Verification items for the finished model (mm, model axes). A direction names the side the tool comes from. Coordinates: 2 decimals unless noted, no trailing zeros. Order: outer loops, then holes, each group sorted by start corner. A loop starts at its lowest first (then second) coordinate and runs counter-clockwise, first axis right, second up.
Q1. Thickness scan on line 1 (Z direction, x = -11, y = 29.5); line 2 (Z direction, x = 8.5, y = -4); line 3 (Y direction, x = 0, z = 23). Record the ranges inside material, lowest first.
Q2. Cross-section at B-B, the plane z = 15. Record the boundary of the cut face in (x, y), and give its area (3 significant figures).
Q3. Set-up check for faces 1 (the flat face through (2, 5, -4)), 2 (the cylindrical face through (-42.15, -41.99, 16.78)): record each of +Z, -Z, +X, -X, +Y, -Y from which the full face is reachable in a straight line by a thin tool's end or side.
Q4. Depth check by flat-ended pin: P1, Ø13, axis at x = 0, y = 0, coming from the -Z side; P2, Ø12, axis at y = -24.5, z = -19.5, coming from the +X side; P3, Ø8, axis at y = 7.5, z = -5.5, coming from the -X side. Enter the tip coordinate at first touch or a pass-through.
Q5. Draft check along Y on faces 3 (the flat face through (0, 45, 16)), 4 (the cylindrical face through (-1.08, -4.88, 16.32)), 5 (the flat face through (-1, 21, 0)). Enter one of: pulls with the +Y half, pulls with the -Y half, needs draft (parallel to the pull), parting line crosses it, or undercut.
Q6. Cross-section at C-C, the plane x = 0. Record the boundary of the cut face in (y, z), and give its area (3 significant figures).
Q7. Cross-section at D-D, the plane y = 0. Record the boundary of the cut face in (x, z).
Q8. Cross-section at A-A, the plane y = 32. Record the boundary of the cut face in (x, z).
from build123d import *

# Parameters (mm, degrees)
SKETCH1_W                               = 40
SKETCH1_H                               = 19.3
SKETCH2_R                               = 20
BOSS_EXTRUDE1_DEPTH                     = 6.5
CBORE_FOR_M8_HEX_HEAD_BOLT1_D           = 10
CBORE_FOR_M8_HEX_HEAD_BOLT1_CBORE_D     = 20
CBORE_FOR_M8_HEX_HEAD_BOLT1_CBORE_DEPTH = 4
F_5_0_5_DIAMETER_HOLE1_D                = 5
F_5_0_5_DIAMETER_HOLE1_DEPTH            = 8
SKETCH7_W                               = 90
SKETCH7_H                               = 90
SKETCH7_R                               = 5
BOSS_EXTRUDE2_DEPTH                     = 33.1
FILLET1_R                               = 10


with BuildPart() as part:
    # Sketch1 → Revolve1 (revolve)
    with BuildSketch(Plane.XZ, mode=Mode.PRIVATE) as revolve1_sk:
        with Locations((20, -16.15)):
            Rectangle(SKETCH1_W, SKETCH1_H)
    revolve(revolve1_sk.sketch.rotate(Axis((0, 0, -6.5), (0, 0, -1)), 270), axis=Axis((0, 0, -6.5), (0, 0, -1)))

    # Sketch2 → Boss-Extrude1 (add)
    with BuildSketch(Plane.XY.offset(-6.5)):
        Circle(SKETCH2_R)
    extrude(amount=BOSS_EXTRUDE1_DEPTH)

    # CBORE for M8 Hex Head Bolt1 (through all)
    with Locations(Plane.XY):
        with Locations((0, 0)):
            CounterBoreHole(CBORE_FOR_M8_HEX_HEAD_BOLT1_D / 2, CBORE_FOR_M8_HEX_HEAD_BOLT1_CBORE_D / 2, CBORE_FOR_M8_HEX_HEAD_BOLT1_CBORE_DEPTH)

    # Ø5.0 (5) Diameter Hole1
    with Locations(Plane.XY):
        with Locations((-15.75, 0), (-11.136931804, 11.136931804), (-11.136931804, -11.136931804), (11.136931804, -11.136931804), (11.136931804, 11.136931804)):
            Hole(F_5_0_5_DIAMETER_HOLE1_D / 2, depth=F_5_0_5_DIAMETER_HOLE1_DEPTH)

    # Sketch7 → Boss-Extrude2 (add)
    with BuildSketch(Plane.XY):
        Rectangle(SKETCH7_W, SKETCH7_H)
        Circle(SKETCH7_R, mode=Mode.SUBTRACT)
    extrude(amount=BOSS_EXTRUDE2_DEPTH)

    # Fillet1
    fillet1_edges = [part.edges().sort_by_distance(p)[0] for p in [
        (45, -45, 16.55),
        (45, 45, 16.55),
        (-45, 45, 16.55),
        (-45, -45, 16.55),
    ]]
    fillet(fillet1_edges, radius=FILLET1_R)


solid = part.part
Check values:
1. line 1: z = -25.8 to -6.5, 0 to 33.1
1. line 2: z = -25.8 to -4, 0 to 33.1
1. line 3: y = -45 to -5, 5 to 45
2. outline: (-45, -35) arc R10 ccw to (-35, -45) - (35, -45) arc R10 ccw to (45, -35) - (45, 35) arc R10 ccw to (35, 45) - (-35, 45) arc R10 ccw to (-45, 35) - close; hole circle Ø10 at (0, 0)
2. area: 7,940 mm2
3. face 1: none
3. face 2: +Z, -Z, -X, -Y
4. P1: stops at z = -25.8
4. P2: stops at x = 35.46
4. P3: stops at x = -39.84
5. face 3: pulls with the +Y half
5. face 4: undercut
5. face 5: needs draft
6. outline: (-45, 0) - (-20, 0) - (-20, -6.5) - (-40, -6.5) - (-40, -25.8) - (-5, -25.8) - (-5, -4) - (-10, -4) - (-10, 0) - (-5, 0) - (-5, 33.1) - (-45, 33.1) - close; (5, -25.8) - (40, -25.8) - (40, -6.5) - (20, -6.5) - (20, 0) - (45, 0) - (45, 33.1) - (5, 33.1) - (5, 0) - (10, 0) - (10, -4) - (5, -4) - close
6. area: 4,150 mm2
7. outline: (-45, 0) - (-20, 0) - (-20, -6.5) - (-40, -6.5) - (-40, -25.8) - (-5, -25.8) - (-5, -4) - (-10, -4) - (-10, 0) - (-5, 0) - (-5, 33.1) - (-45, 33.1) - close; (5, -25.8) - (40, -25.8) - (40, -6.5) - (20, -6.5) - (20, 0) - (45, 0) - (45, 33.1) - (5, 33.1) - (5, 0) - (10, 0) - (10, -4) - (5, -4) - close; hole (-18.25, -8) - (-13.25, -8) - (-13.25, 0) - (-18.25, 0) - close
8. outline: (-45, 0) - (45, 0) - (45, 33.1) - (-45, 33.1) - close; (-24, -25.8) - (24, -25.8) - (24, -6.5) - (-24, -6.5) - close
